Geometry: final body of the model. Coordinates: model frame, mm. Face numbers are marked on the shaded views. A direction names the side the tool comes from. Coordinates: 2 decimals unless noted, no trailing zeros. Loops run counter-clockwise (first coordinate to the right, second up) from the corner with the lowest first, then second, coordinate; pieces in that order, holes last. Notation, with made-up numbers: (-7.75, 44) - (43.25, 44) arc R12 cw to (43.25, 59) - close; hole circle Ø1 at (13.5, 43.5). An arc over 180 degrees is marked (long way). Put each result on its own line as item: value. Start each with the question number.
1) Section C-C on x = 20.5. Output: boundary loops of the cut face in (y, z), and give its area (3 significant figures).
2) Contact query for flat-ended pins moving along their axis: pin 1 Ø9 at (x, y) = (10.5, 37) entering from +Z; pin 2 Ø5 at (x, y) = (16, 32) entering from +Z; pin 3 Ø8 at (x, y) = (14.5, 27.5) entering from +Z. Output: stop coordinate, or through.
3) Material intervals for line 1 along X through (y, z) = (24.5, -10) (3 decimals); line 2 along Z through (x, y) = (2.25, 41); line 3 along Y through (x, z) = (8, 2), sorted ascending. Write a range as from..to.
4) Draft query along X for the marked faces 3, 4 and 5. Return one class per face: +X half, -X half, draft (parallel to the pull), parting line (faces both ways), or undercut.
5) Section B-B on z = -12. Output: boundary loops of the cut face in (x, y) (3 decimals).
6) Section D-D on x = 8.75. Output: boundary loops of the cut face in (y, z), and give its area (3 significant figures).
7) Section A-A on y = 32.75. Output: boundary loops of the cut face in (x, z) (3 decimals).
8) Reachability of the marked faces 1 and 2 from +Z, -Z, +X, -X, +Y, -Y: full face, straight path, thin tool, end or side. Return the list, or none.
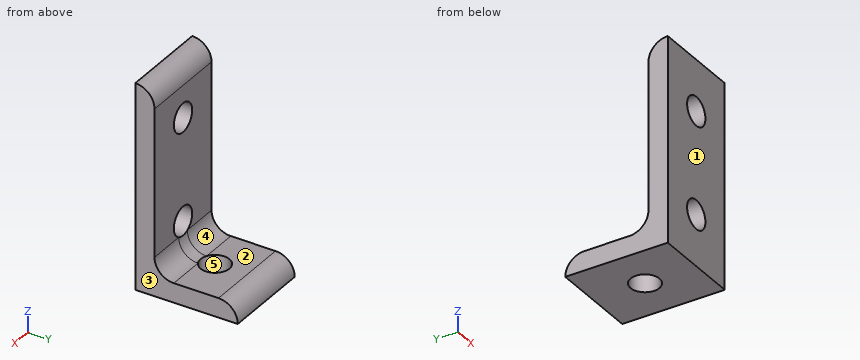
```python
from build123d import *

# Parameters (mm, degrees)
EXTRUDE1_DEPTH     = 22.225
SKETCH2_R          = 3.5687
CUT_EXTRUDE1_DEPTH = 5.7752
FILLET1_R          = 4.7752
CUT_EXTRUDE2_DEPTH = 23.225


with BuildPart() as part:
    # Sketch1 → Extrude1 (new body)
    with BuildSketch(Plane(origin=(0, 0, 0), x_dir=(0, 0, -1), z_dir=(1, 0, 0))):
        with BuildLine():
            Line((-28.199163803, 21.897674685), (22.600836197, 21.897674685))
            Line((22.600836197, 21.897674685), (17.825636197, 26.672874685))
            Line((17.825636197, 26.672874685), (-23.423963803, 26.672874685))
            ThreePointArc((-23.423963803, 26.672874685), (-26.800540105, 25.274250987), (-28.199163803, 21.897674685))
        make_face()
    extrude(amount=EXTRUDE1_DEPTH)

    # Sketch2 → Cut-Extrude1 (cut, through all)
    with BuildSketch(Plane(origin=(0, 26.672874685, 0), x_dir=(1, 0, 0), z_dir=(0, 1, 0))):
        with Locations((11.1125, -15.499163803)):
            Circle(SKETCH2_R)
        with Locations((11.1125, 9.900836197)):
            Circle(SKETCH2_R)
    extrude(amount=-CUT_EXTRUDE1_DEPTH, mode=Mode.SUBTRACT)

    # Mirror1: part across plane


with BuildPart() as part_1:
    add(part.part)
    add(part.part.mirror(Plane(origin=(22.225, 21.897674685, -22.600836197), x_dir=(0, 0.707106781, 0.707106781), z_dir=(0, -0.707106781, 0.707106781))))

    # Fillet1
    fillet1_edges = [part_1.edges().sort_by_distance(p)[0] for p in [
        (11.1125, 26.672874685, -17.825636197),
    ]]
    fillet(fillet1_edges, radius=FILLET1_R)

    # Sketch3 → Cut-Extrude2 (cut, through all)
    with BuildSketch(Plane(origin=(22.225, 0, 0), x_dir=(0, 0, -1), z_dir=(1, 0, 0))):
        with BuildLine():
            Line((17.825636197, 67.922474685), (17.825636197, 42.522474685))
            ThreePointArc((17.825636197, 42.522474685), (19.224259895, 45.899050987), (22.600836197, 47.297674685))
            Line((22.600836197, 47.297674685), (22.600836197, 72.697674685))
            ThreePointArc((22.600836197, 72.697674685), (19.224259895, 71.299050987), (17.825636197, 67.922474685))
        make_face()
    extrude(amount=-CUT_EXTRUDE2_DEPTH, mode=Mode.SUBTRACT)


solid = part_1.part
```
Answer block:
1. outline: (21.9, -22.6) - (47.3, -22.6) arc R4.78 ccw to (42.52, -17.83) - (31.45, -17.83) arc R4.78 cw to (26.67, -13.05) - (26.67, 23.42) arc R4.78 ccw to (21.9, 28.2) - close
1. area: 336 mm²
2. pin 1: stops at z = -17.83
2. pin 2: stops at z = -17.41
2. pin 3: stops at z = 27.92
3. line 1: x = 0..7.545, 14.68..22.225
3. line 2: z = -22.6..-17.83
3. line 3: y = 21.9..26.67
4. face 3: +X half
4. face 4: draft
4. face 5: undercut
5. outline: (0, 21.898) - (8.226, 21.898) - (8.226, 26.673) - (0, 26.673) - close; (13.999, 21.898) - (22.225, 21.898) - (22.225, 26.673) - (13.999, 26.673) - close
6. outline: (21.9, -22.6) - (31.92, -22.6) - (31.92, -17.83) - (31.45, -17.83) arc R4.78 cw to (26.67, -13.05) - (26.67, -12.58) - (21.9, -12.58) - close; (21.9, -7.23) - (26.67, -7.23) - (26.67, 12.82) - (21.9, 12.82) - close; (21.9, 18.17) - (26.67, 18.17) - (26.67, 23.42) arc R4.78 ccw to (21.9, 28.2) - close; (37.27, -22.6) - (47.3, -22.6) arc R4.78 ccw to (42.52, -17.83) - (37.27, -17.83) - close
6. area: 260 mm²
7. outline: (0, -22.601) - (8.059, -22.601) - (8.059, -17.826) - (0, -17.826) - close; (14.166, -22.601) - (22.225, -22.601) - (22.225, -17.826) - (14.166, -17.826) - close
8. face 1: +Z, -Z, +X, -X, -Y
8. face 2: +Z, +X, -X, +Y
